```python
from build123d import *

# Parameters (mm, degrees)
SKETCH_1_W               = 344
SKETCH_1_H               = 420
SKETCH_1_R               = 1.6
EXTRUDE_1_DEPTH          = 2
CUT_EXTRUDE_1_DEPTH      = 272.455337026
CUT_EXTRUDE_1_DEPTH_BACK = 272.455337026
SKETCH_2_W               = 50
SKETCH_2_H               = 27.5
FILLET_1_R               = 10


with BuildPart() as part:
    # 草图1 → 凸台-拉伸1 (new, symmetric)
    with BuildSketch(Plane(origin=(0, 0, 0), x_dir=(1, 0, 0), z_dir=(0, 1, 0))):
        Rectangle(SKETCH_1_W, SKETCH_1_H)
        with Locations(Location((-167, -170, 0), (0, 0, 270))):
            Circle(SKETCH_1_R, mode=Mode.SUBTRACT)
        with Locations(Location((167, -170, 0), (0, 0, 270))):
            Circle(SKETCH_1_R, mode=Mode.SUBTRACT)
        with Locations(Location((-167, -100, 0), (0, 0, 270))):
            Circle(SKETCH_1_R, mode=Mode.SUBTRACT)
        with Locations(Location((-167, -30, 0), (0, 0, 270))):
            Circle(SKETCH_1_R, mode=Mode.SUBTRACT)
        with Locations(Location((-167, 40, 0), (0, 0, 270))):
            Circle(SKETCH_1_R, mode=Mode.SUBTRACT)
        with Locations(Location((-167, 110, 0), (0, 0, 270))):
            Circle(SKETCH_1_R, mode=Mode.SUBTRACT)
        with Locations(Location((-167, 180, 0), (0, 0, 270))):
            Circle(SKETCH_1_R, mode=Mode.SUBTRACT)
        with Locations(Location((167, -100, 0), (0, 0, 270))):
            Circle(SKETCH_1_R, mode=Mode.SUBTRACT)
        with Locations(Location((167, -30, 0), (0, 0, 270))):
            Circle(SKETCH_1_R, mode=Mode.SUBTRACT)
        with Locations(Location((167, 40, 0), (0, 0, 270))):
            Circle(SKETCH_1_R, mode=Mode.SUBTRACT)
        with Locations(Location((167, 110, 0), (0, 0, 270))):
            Circle(SKETCH_1_R, mode=Mode.SUBTRACT)
        with Locations(Location((167, 180, 0), (0, 0, 270))):
            Circle(SKETCH_1_R, mode=Mode.SUBTRACT)
    extrude(amount=EXTRUDE_1_DEPTH, both=True)

    # 草图2 → 切除-拉伸1 (cut, two sides: drawn at the far end of the back side and taken through both)
    with BuildSketch(Plane(origin=(0, 0, 0), x_dir=(1, 0, 0), z_dir=(0, 1, 0)).offset(-CUT_EXTRUDE_1_DEPTH_BACK)):
        with Locations((0, -196.25)):
            Rectangle(SKETCH_2_W, SKETCH_2_H)
    extrude(amount=CUT_EXTRUDE_1_DEPTH + CUT_EXTRUDE_1_DEPTH_BACK, mode=Mode.SUBTRACT)

    # 圆角1
    fillet_1_edges = [part.edges().sort_by_distance(p)[0] for p in [
        (-172, 0, -210),
        (172, 0, -210),
        (172, 0, 210),
        (-172, 0, 210),
    ]]
    fillet(fillet_1_edges, radius=FILLET_1_R)


solid = part.part
```
Geometry check sheet. Reference: the model listing, model coordinates, mm. Give positions to 0.01 mm unless a question says otherwise; leave off trailing zeros. Write each loop counter-clockwise with the first axis right and the second up, starting at its lowest first coordinate (ties: lowest second). Pieces come first, ordered by that corner, then holes.
1) Material ranges on L1, parallel to X at y = 1.15, z = 30; L2, parallel to Z at x = -7, y = 0.55, recorded low to high.
2) Section check A-A, the plane x = 1. Record the boundary of the cut face in (y, z), and give its area (3 significant figures).
3) Gauge pin test, flat ends, axial feed: pin 1 (1.5 mm diameter, centred on x = 19, y = -1, fed in from +Z); pin 2 (1.9 mm diameter, centred on x = 167, z = 170, fed in from -Y); pin 3 (5 mm diameter, centred on x = 167, z = -40, fed in from +Y). Record the tip position at first contact, or that the pin passes through.
Computed:
1. L1: x = -172 to -168.6, -165.4 to 165.4, 168.6 to 172
1. L2: z = -210 to 182.5
2. outline: (-2, -210) - (2, -210) - (2, 182.5) - (-2, 182.5) - close
2. area: 1,570 mm2
3. pin 1: stops at z = 182.5
3. pin 2: passes through
3. pin 3: stops at y = 2
